Geometry: final body of the model. Coordinates: model frame, mm. Give positions to 0.01 mm unless a question says otherwise; leave off trailing zeros. Loops run counter-clockwise (first coordinate to the right, second up) from the corner with the lowest first, then second, coordinate; pieces in that order, holes last.
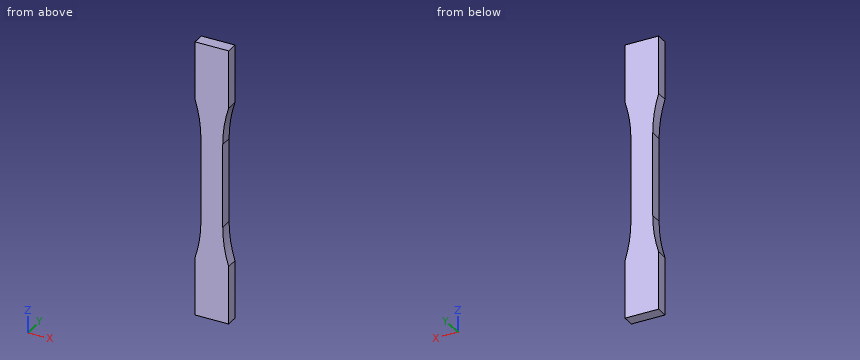
Autodesk Inventor part; units mm, degrees
ref_plane "YZ Plane" through (0, 0, 0) normal (1, 0, 0) x (0, 1, 0)
ref_plane "XZ Plane" through (0, 0, 0) normal (0, 1, 0) x (-1, 0, 0)
ref_plane "XY Plane" through (0, 0, 0) normal (0, 0, 1) x (1, 0, 0)
sketch "Sketch1" plane through (0, 0, 0) normal (0, 1, 0) x (-1, 0, 0)
  line L0 (0, 0) -> (20, 0)
  line L1 (3.5, 57.5) -> (3.5, 82.5)
  line L2 (16.5, 57.5) -> (16.5, 82.5)
  arc A0 (16.5, 57.5) -> (20, 34.702) centre (92.5, 57.5) ccw
  arc A1 (0, 34.702) -> (3.5, 57.5) centre (-72.5, 57.5) ccw
  line L3 (3.5, 82.5) -> (16.5, 82.5) construction
  line L4 (0, 34.702) -> (0, 0)
  line L5 (20, 34.702) -> (20, 0)
  line L6 (0, 165) -> (20, 165)
  line L7 (3.5, 107.5) -> (3.5, 82.5)
  line L8 (16.5, 107.5) -> (16.5, 82.5)
  arc A2 (20, 130.298) -> (16.5, 107.5) centre (92.5, 107.5) ccw
  arc A3 (3.5, 107.5) -> (0, 130.298) centre (-72.5, 107.5) ccw
  line L9 (0, 130.298) -> (0, 165)
  line L10 (20, 130.298) -> (20, 165)
  dimension "d2" = 20
  dimension "d5" = 76
  dimension "d6" = 76
  dimension "d7" = 82.5
  dimension "d8" = 13
  dimension "d9" = 25
extrude "Extrusion1" add sketch "Sketch1" along normal blind 7
properties part number "ASTM D638-10-1"
Item 1: Ray query, probe 1 along X at (y, z) = (2, 104.5); probe 2 along X at (y, z) = (5, 36). Return the intervals inside material, ascending.
Values follow:
probe 1: x = -16.5 to -3.5
probe 2: x = -19.6 to -0.4
Item 2: Section query B-B on z = 61. Return loops of the section in (x, y), plus the area to 3 significant figures.
Values follow:
outline: (-16.5, 0) - (-3.5, 0) - (-3.5, 7) - (-16.5, 7) - close
area: 91.0 mm2
Item 3: Section query C-C on z = 122. Return loops of the section in (x, y), plus the area to 3 significant figures.
Values follow:
outline: (-17.9, 0) - (-2.1, 0) - (-2.1, 7) - (-17.9, 7) - close
area: 111 mm2
Item 4: Section query A-A on y = 1.5. Return loops of the section in (x, z), plus the area to 3 significant figures.
Values follow:
outline: (-20, 0) - (0, 0) - (0, 34.7) arc R76 cw to (-3.5, 57.5) - (-3.5, 107.5) arc R76 cw to (0, 130.3) - (0, 165) - (-20, 165) - (-20, 130.3) arc R76 cw to (-16.5, 107.5) - (-16.5, 57.5) arc R76 cw to (-20, 34.7) - close
area: 2,740 mm2
Item 5: Pin query (flat end, axial travel): pin 1 (1 mm diameter, centred on y = 3.5, z = 55, fed in from -X). Return the tip coordinate at first contact, or that it passes through.
Values follow:
pin 1: stops at x = -16.56
